Verification items for this drawing (mm, ordinates from the low corner). A direction names the side the tool comes from. Give positions to 0.01 mm unless a question says otherwise; leave off trailing zeros. Order: outer loops, then holes, each group sorted by start corner. A loop starts at its lowest first (then second) coordinate and runs counter-clockwise, first axis right, second up. Notation, with made-up numbers: M 66,-5 L 84,-5 A22 cw 84,26 Z; hole C -19.75,-17.5 d8. An arc over 180 degrees is marked long. Answer as a JSON object with one key per item and string values.
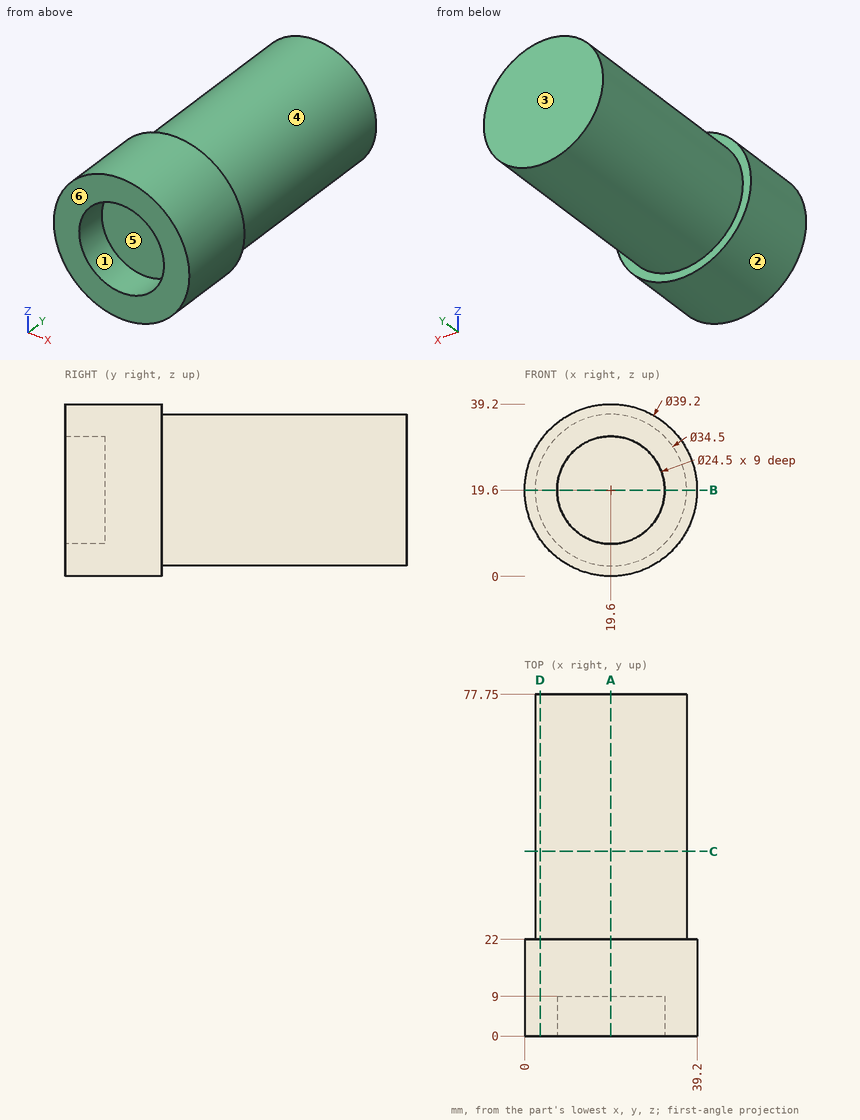
Q1. Section check A-A on x = 19.6. Record the cut outline in (y, z).
Resolved:
{"outline": "M 0,0 L 22,0 L 22,2.35 L 77.75,2.35 L 77.75,36.85 L 22,36.85 L 22,39.2 L 0,39.2 L 0,31.85 L 9,31.85 L 9,7.35 L 0,7.35 Z"}
Q2. Release check for a two-part mould opening along Z. For the marked faces 1, 2 and 3 record: +Z half, -Z half, draft (parallel to the pull), parting line (faces both ways), or undercut.
Resolved:
{"face 1": "undercut", "face 2": "parting line", "face 3": "draft"}
Q3. Material ranges on L1, parallel to X at y = 4.5, z = 19.6; L2, parallel to Z at x = 19, y = 6; L3, parallel to Y at x = 4, z = 29.5, recorded low to high.
Resolved:
{"L1": "x = 0 to 7.35, 31.85 to 39.2", "L2": "z = 0.01 to 7.36, 31.84 to 39.19", "L3": "y = 0 to 22"}
Q4. Section check C-C on y = 42. Record the cut outline in (x, z).
Resolved:
{"outline": "C 19.6,19.6 d34.5"}
Q5. Tool access check on the marked faces 4, 5 and 6. Record the directions out of +Z, -Z, +X, -X, +Y, -Y that give a thin tool (end or side, any length) a straight path to the whole face; none if there is none.
Resolved:
{"face 4": "+Y", "face 5": "-Y", "face 6": "+Z, -Z, +X, -X, -Y"}
Q6. Gauge pin test, flat ends, axial feed: pin 1 Ø5 at (y, z) = (57, 21.5) entering from +X; pin 2 Ø5 at (y, z) = (11.5, 25) entering from -X; pin 3 Ø6 at (x, y) = (21, 31.5) entering from +Z. Record the tip position at first contact, or that the pin passes through.
Resolved:
{"pin 1": "stops at x = 36.85", "pin 2": "stops at x = 0.22", "pin 3": "stops at z = 36.85"}
Q7. Section check D-D on x = 3.5. Record the cut outline in (y, z).
Resolved:
{"outline": "M 0,8.42 L 22,8.42 L 22,13.41 L 77.75,13.41 L 77.75,25.79 L 22,25.79 L 22,30.78 L 0,30.78 Z"}
Q8. Section check B-B on z = 19.6. Record the cut outline in (x, y).
Resolved:
{"outline": "M 0,0 L 7.35,0 L 7.35,9 L 31.85,9 L 31.85,0 L 39.2,0 L 39.2,22 L 36.85,22 L 36.85,77.75 L 2.35,77.75 L 2.35,22 L 0,22 Z"}
